from build123d import *

# Parameters (mm, degrees)
F0_W     = 3.175
F0_H     = 50.7914833724
F1_DEPTH = 50.8
F3_DEPTH = 3.176
F4_DEPTH = 3.175
F5_DEPTH = 3.175
F6_W     = 3.175
F6_H     = 50.7914833724
F7_DEPTH = 6.35
F8_R     = 1.5875
F9_DEPTH = 63.5


with BuildPart() as f1:
    # F0 (on Right) → F1 (new body)
    with BuildSketch(Plane.YZ):
        with Locations((1.5875, 25.3957416862)):
            Rectangle(F0_W, F0_H)
    extrude(amount=F1_DEPTH)

    # F2 (on face) → F3 (cut, through all)
    with BuildSketch(Plane.XZ):
        with BuildLine():
            Line((40.64, 38.1), (10.16, 38.1))
            ThreePointArc((10.16, 38.1), (9.0374679849, 37.6350320151), (8.5725, 36.5125))
            Line((8.5725, 36.5125), (8.5725, 23.8125))
            ThreePointArc((8.5725, 23.8125), (9.0374679849, 22.6899679849), (10.16, 22.225))
            Line((10.16, 22.225), (40.64, 22.225))
            ThreePointArc((40.64, 22.225), (41.7625320151, 22.6899679849), (42.2275, 23.8125))
            Line((42.2275, 23.8125), (42.2275, 36.5125))
            ThreePointArc((42.2275, 36.5125), (41.7625320151, 37.6350320151), (40.64, 38.1))
        make_face()
    extrude(amount=-F3_DEPTH, mode=Mode.SUBTRACT)

    # F4 (add): a face of the model
    f4_faces = [f1.faces().sort_by_distance(p)[0] for p in [
        (0, 1.5875, 25.3957416862),
    ]]
    extrude(f4_faces, amount=F4_DEPTH)

    # F5 (add): a face of the model
    f5_faces = [f1.faces().sort_by_distance(p)[0] for p in [
        (50.8, 1.5875, 25.3957416862),
    ]]
    extrude(f5_faces, amount=F5_DEPTH)

    # F6 (on face) → F7 (join)
    with BuildSketch(Plane.XZ):
        with Locations((-1.5875, 25.3957416862)):
            Rectangle(F6_W, F6_H)
        with Locations((52.3875, 25.3957416862)):
            Rectangle(F6_W, F6_H)
    extrude(amount=F7_DEPTH)

    # F8 (on face) → F9 (cut)
    with BuildSketch(Plane.YZ.offset(53.975)):
        with Locations((-3.175, 47.6164833724)):
            Circle(F8_R)
        with Locations((-3.175, 3.175)):
            Circle(F8_R)
    extrude(amount=-F9_DEPTH, mode=Mode.SUBTRACT)


solid = f1.part
Build history of the part. All positions in model axes, mm. A direction names the side the tool comes from. Coordinates: 2 decimals unless noted, no trailing zeros. Write each loop counter-clockwise with the first axis right and the second up, starting at its lowest first coordinate (ties: lowest second). Pieces come first, ordered by that corner, then holes.
(1) 3-axis set-ups, long thin cutter, end or side, ignore diameter. For faces 1 (the cylindrical face through (-1.565, -3.519, 46.067)), 2 (the flat face through (25, 0, 19)), 3 (the flat face through (25, 2, 22.225)): which of +Z, -Z, +X, -X, +Y, -Y reach the whole face in a straight line?
(2) Cut at B-B on x = 21.5. List the corners of the cut face in (y, z) (3 decimals), and give its area (3 significant figures).
(3) Cut at C-C on y = 1. List the corners of the cut face in (x, z) (1 decimal), and give its area (3 significant figures).
(4) Mould opens along Z. For faces 4 (the cylindrical face through (52.4, -2.3, 4.5)), 5 (the flat face through (-2, -6.35, 26)), 6 (the flat face through (19, 1, 0)) say: pulls with the +Z half, pulls with the -Z half, needs draft (parallel to the pull), parting line crosses it, or undercut.
(5) Cut at D-D on z = 20. List the corners of the cut face in (x, y) (3 decimals).
(6) Drill centre lines: line 1 (X direction, y = -3.5, z = 26.5) (3 decimals); line 2 (Z direction, x = 32, y = 1.25) (3 decimals); line 3 (X direction, y = 2.75, z = 27.5) (1 decimal). Where is each one in solid material? Low to high.
(7) Pin check, flat tips, straight feed: pin 1 Ø1.5 at (x, z) = (35.5, 18.5) entering from -Y; pin 2 Ø1.9 at (y, z) = (-3.18, 47.62) entering from +X. Stop position of each tip, or through.
Working result:
1. face 1: +X, -X
1. face 2: +Z, -Z, -Y
1. face 3: +Y, -Y
2. outline: (0, 0) - (3.175, 0) - (3.175, 22.225) - (0, 22.225) - close; (0, 38.1) - (3.175, 38.1) - (3.175, 50.791) - (0, 50.791) - close
2. area: 111 mm2
3. outline: (-3.2, 0) - (54, 0) - (54, 50.8) - (-3.2, 50.8) - close; hole (8.6, 23.8) arc R1.6 ccw to (10.2, 22.2) - (40.6, 22.2) arc R1.6 ccw to (42.2, 23.8) - (42.2, 36.5) arc R1.6 ccw to (40.6, 38.1) - (10.2, 38.1) arc R1.6 ccw to (8.6, 36.5) - close
3. area: 2,370 mm2
4. face 4: undercut
4. face 5: needs draft
4. face 6: pulls with the -Z half
5. outline: (-3.175, -6.35) - (0, -6.35) - (0, 0) - (50.8, 0) - (50.8, -6.35) - (53.975, -6.35) - (53.975, 3.175) - (-3.175, 3.175) - close
6. line 1: x = -3.175 to 0, 50.8 to 53.975
6. line 2: z = 0 to 22.225, 38.1 to 50.791
6. line 3: x = -3.2 to 8.6, 42.2 to 54
7. pin 1: stops at y = 0
7. pin 2: passes through
